Check sheet for the modelled part. Datum: model origin and axes. Units: mm. A direction names the side the tool comes from. Round coordinates to 2 decimals unless told otherwise and drop trailing zeros. Write each loop counter-clockwise with the first axis right and the second up, starting at its lowest first coordinate (ties: lowest second). Pieces come first, ordered by that corner, then holes. Notation, with made-up numbers: M 13.25,20.5 L 34.25,20.5 A30 cw 34.25,52.5 Z; hole C 19,-33 d2. An arc over 180 degrees is marked long. Answer in a Markdown table with one row per item.
```python
from build123d import *

# Parameters (mm, degrees)
F0_W      = 120
F0_H      = 60
F1_DEPTH  = 30
F2_W      = 12
F2_H      = 21.2132
F3_DEPTH  = 8
F4_W      = 114
F4_H      = 54
F5_DEPTH  = 20
F6_W      = 3
F6_H      = 15
F7_DEPTH  = 12
F8_W      = 20
F8_H      = 15
F9_DEPTH  = 3
F10_R     = 5
F11_R     = 5.08
F12_W     = 3
F12_H     = 15
F13_DEPTH = 3
F14_W     = 10
F14_H     = 15
F15_DEPTH = 2


with BuildPart() as f1:
    # F0 (on Top) → F1 (new body)
    with BuildSketch(Plane.XY):
        Rectangle(F0_W, F0_H)
    extrude(amount=F1_DEPTH)

    # F2 (on face) → F3 (cut)
    with BuildSketch(Plane.XY.offset(30)):
        Rectangle(F2_W, F2_H)
    extrude(amount=-F3_DEPTH, mode=Mode.SUBTRACT)

    # F4 (on face) → F5 (cut)
    with BuildSketch(Plane(origin=(0, 0, 0), x_dir=(1, 0, 0), z_dir=(0, 0, -1))):
        Rectangle(F4_W, F4_H)
    extrude(amount=-F5_DEPTH, mode=Mode.SUBTRACT)

    # F6 (on face) → F7 (join)
    with BuildSketch(Plane(origin=(0, 0, 20), x_dir=(1, 0, 0), z_dir=(0, 0, -1))):
        with Locations((-30, 0)):
            Rectangle(F6_W, F6_H)
        with Locations((30, 0)):
            Rectangle(F6_W, F6_H)
    extrude(amount=F7_DEPTH)

    # F8 (on face) → F9 (join)
    with BuildSketch(Plane(origin=(0, 0, 8), x_dir=(1, 0, 0), z_dir=(0, 0, -1))):
        with Locations((-38.5, 0)):
            Rectangle(F8_W, F8_H)
        with Locations((38.5, 0)):
            Rectangle(F8_W, F8_H)
    extrude(amount=F9_DEPTH)

    # F10
    f10_edges = [f1.edges().sort_by_distance(p)[0] for p in [
        (-48.5, -7.5, 6.5),
        (-48.5, 7.5, 6.5),
        (48.5, 7.5, 6.5),
        (48.5, -7.5, 6.5),
    ]]
    fillet(f10_edges, radius=F10_R)

    # F11
    f11_edges = [f1.edges().sort_by_distance(p)[0] for p in [
        (-6, 10.6066, 26),
        (-6, -10.6066, 26),
    ]]
    fillet(f11_edges, radius=F11_R)

    # F12 (on face) → F13 (cut, through all)
    with BuildSketch(Plane(origin=(0, 30, 0), x_dir=(-1, 0, 0), z_dir=(0, 1, 0))):
        with Locations((0, 7.5)):
            Rectangle(F12_W, F12_H)
    extrude(amount=-F13_DEPTH, mode=Mode.SUBTRACT)

    # F14 (on face) → F15 (cut, through all)
    with BuildSketch(Plane.XY.offset(22)):
        with Locations((1, 0.213741)):
            Rectangle(F14_W, F14_H)
    extrude(amount=-F15_DEPTH, mode=Mode.SUBTRACT)


solid = f1.part
```
1. Section check B-B, the plane x = -38.5. Record the cut outline in (y, z), and give its area (3 significant figures).
Found:
| item | result |
|---|---|
| outline | M -30,0 L -27,0 L -27,20 L 27,20 L 27,0 L 30,0 L 30,30 L -30,30 Z; M -7.5,5 L 7.5,5 L 7.5,8 L -7.5,8 Z |
| area | 765 mm2 |
2. Section check C-C, the plane z = 13.5. Record the cut outline in (x, y), and give its area (4 significant figures).
Found:
| item | result |
|---|---|
| outline | M -60,-30 L 60,-30 L 60,30 L 1.5,30 L 1.5,27 L 57,27 L 57,-27 L -57,-27 L -57,27 L -1.5,27 L -1.5,30 L -60,30 Z; M -31.5,-7.5 L -28.5,-7.5 L -28.5,7.5 L -31.5,7.5 Z; M 28.5,-7.5 L 31.5,-7.5 L 31.5,7.5 L 28.5,7.5 Z |
| area | 1,125 mm2 |
3. Go/stop test with flat-tipped pins: pin 1 (3 mm diameter, centred on x = -14, y = -4, fed in from -Z); pin 2 (16.5 mm diameter, centred on x = -41, y = 0.5, fed in from -Z); pin 3 (13 mm diameter, centred on x = 2, y = 1.5, fed in from +Z). Record where each tip stops, or that it passes through.
Found:
| item | result |
|---|---|
| pin 1 | stops at z = 20 |
| pin 2 | stops at z = 5 |
| pin 3 | stops at z = 30 |
4. Scan lines: L1, parallel to X at y = -6.5, z = 10.5; L2, parallel to Y at x = -5.5, z = 18.25; L3, parallel to X at y = -18, z = 9.5. Record each from-to range of solid material in increasing order.
Found:
| item | result |
|---|---|
| L1 | x = -60 to -57, -31.5 to -28.5, 28.5 to 31.5, 57 to 60 |
| L2 | y = -30 to -27, 27 to 30 |
| L3 | x = -60 to -57, 57 to 60 |
5. Section check A-A, the plane z = 18.5. Record the cut outline in (x, y), and give its area (3 significant figures).
Found:
| item | result |
|---|---|
| outline | M -60,-30 L 60,-30 L 60,30 L -60,30 Z; M -31.5,-7.5 L -28.5,-7.5 L -28.5,7.5 L -31.5,7.5 Z; M 28.5,-7.5 L 31.5,-7.5 L 31.5,7.5 L 28.5,7.5 Z; hole M -57,-27 L 57,-27 L 57,27 L -57,27 Z |
| area | 1,130 mm2 |
6. Access from +Z, -Z, +X, -X, +Y, -Y to the whole of each face (thin tool, end or side, straight path). Record for faces 1 (the face through (-31.5, 0, 14)), 2 (the face through (2, 10.607, 26)), 3 (the face through (28.5, 0, 13)).
Found:
| item | result |
|---|---|
| face 1 | none |
| face 2 | +Z |
| face 3 | -Z |
7. Section check D-D, the plane x = 22. Record the cut outline in (y, z), and give its area (3 significant figures).
Found:
| item | result |
|---|---|
| outline | M -30,0 L -27,0 L -27,20 L 27,20 L 27,0 L 30,0 L 30,30 L -30,30 Z |
| area | 720 mm2 |
